from build123d import *

# Parameters (mm, degrees)
F0_R     = 2.54
F1_DEPTH = 5.08
F2_R     = 2.54
F3_R     = 2.53999


# Not quite as in the source:
# - a fillet or chamfer is up to 0.001 mm smaller than in the source, because OpenCascade refuses the exact size


with BuildPart() as f1:
    # F0 (on Front) → F1 (new body)
    with BuildSketch(Plane.XZ):
        Circle(F0_R)
    extrude(amount=F1_DEPTH)

    # F2
    f2_edges = [f1.edges().sort_by_distance(p)[0] for p in [
        (-2.54, -5.08, 0),
    ]]
    fillet(f2_edges, radius=F2_R)

    # F3 (radius 2.54 in the source; OpenCascade refuses exactly that, so slightly less here)
    f3_edges = [f1.edges().sort_by_distance(p)[0] for p in [
        (-2.54, 0, 0),
    ]]
    fillet(f3_edges, radius=F3_R)


solid = f1.part
Read the model definition and answer for the solid it produces. Units are mm, in the model's axes. Round coordinates to 2 decimals unless told otherwise and drop trailing zeros. Write each loop counter-clockwise with the first axis right and the second up, starting at its lowest first coordinate (ties: lowest second). Pieces come first, ordered by that corner, then holes.
1. A straight line is drawn through the part: L1, parallel to Y at x = -1.1, z = 0.75. Find the intervals that lie inside material, in ascending order.
2. Given pin 1 Ø3 at (y, z) = (-2, 2) entering from +X; pin 2 Ø1.5 at (x, y) = (-0.5, -4) entering from -Z; pin 3 Ø2 at (y, z) = (-4.5, -1) entering from -X, each flat-ended and moving along its own axis, determine where each tip first touches the part or whether it passes through.
3. The part is cut by section A-A, the plane y = -4.1. Determine the outline of the cut face in (x, z).
Values:
1. L1: y = -4.7 to -0.38
2. pin 1: stops at x = 2.47
2. pin 2: stops at z = -2.41
2. pin 3: stops at x = -2.24
3. outline: circle Ø4.01 at (0, 0)
